The listing builds one solid part. Answer for the finished solid, in the listing's coordinates (mm). Face numbers are marked on the shaded views. Coordinates: 2 decimals unless noted, no trailing zeros. Order: outer loops, then holes, each group sorted by start corner. A loop starts at its lowest first (then second) coordinate and runs counter-clockwise, first axis right, second up.
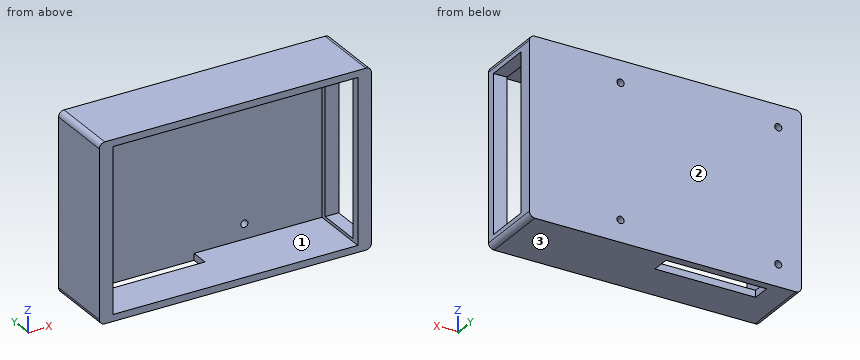
from build123d import *

# Parameters (mm, degrees)
SKETCH1_W           = 100
SKETCH1_H           = 65
BOSS_EXTRUDE2_DEPTH = 25
SKETCH1_5_W         = 90
SKETCH1_5_H         = 60
CUT_EXTRUDE1_DEPTH  = 22
SKETCH3_R           = 1.3
CUT_EXTRUDE2_DEPTH  = 18
FILLET2_R           = 2
FILLET3_R           = 2
FILLET4_R           = 2
FILLET5_R           = 2
SKETCH5_W           = 37
SKETCH5_H           = 6.720639237
CUT_EXTRUDE3_DEPTH  = 10
SKETCH6_W           = 57.574734681
SKETCH6_H           = 17
CUT_EXTRUDE4_DEPTH  = 10


with BuildPart() as part:
    # Sketch1 → Boss-Extrude2 (new body)
    with BuildSketch(Plane(origin=(0, 0, 0), x_dir=(1, 0, 0), z_dir=(0, 1, 0))):
        Rectangle(SKETCH1_W, SKETCH1_H)
    extrude(amount=BOSS_EXTRUDE2_DEPTH)

    # Sketch1_5 → Cut-Extrude1 (cut)
    with BuildSketch(Plane(origin=(0, 0, 0), x_dir=(1, 0, 0), z_dir=(0, 1, 0))):
        Rectangle(SKETCH1_5_W, SKETCH1_5_H)
    extrude(amount=CUT_EXTRUDE1_DEPTH, mode=Mode.SUBTRACT)

    # Sketch3 → Cut-Extrude2 (cut)
    with BuildSketch(Plane.XZ.offset(-22)):
        with Locations(Location((-41.5, 24.5, 0), (0, 0, 270))):
            Circle(SKETCH3_R)
        with Locations(Location((-41.5, -24.5, 0), (0, 0, 270))):
            Circle(SKETCH3_R)
        with Locations(Location((16.5, -24.5, 0), (0, 0, 270))):
            Circle(SKETCH3_R)
        with Locations(Location((16.5, 24.5, 0), (0, 0, 270))):
            Circle(SKETCH3_R)
    extrude(amount=-CUT_EXTRUDE2_DEPTH, mode=Mode.SUBTRACT)

    # Fillet2
    fillet2_edges = [part.edges().sort_by_distance(p)[0] for p in [
        (50, 12.5, 32.5),
    ]]
    fillet(fillet2_edges, radius=FILLET2_R)

    # Fillet3
    fillet3_edges = [part.edges().sort_by_distance(p)[0] for p in [
        (-50, 12.5, 32.5),
    ]]
    fillet(fillet3_edges, radius=FILLET3_R)

    # Fillet4
    fillet4_edges = [part.edges().sort_by_distance(p)[0] for p in [
        (-50, 12.5, -32.5),
    ]]
    fillet(fillet4_edges, radius=FILLET4_R)

    # Fillet5
    fillet5_edges = [part.edges().sort_by_distance(p)[0] for p in [
        (50, 12.5, -32.5),
    ]]
    fillet(fillet5_edges, radius=FILLET5_R)

    # Sketch5 → Cut-Extrude3 (cut)
    with BuildSketch(Plane(origin=(0, 0, -32.5), x_dir=(-1, 0, 0), z_dir=(0, 0, -1))):
        with Locations((20.5, 18.639680381)):
            Rectangle(SKETCH5_W, SKETCH5_H)
    extrude(amount=-CUT_EXTRUDE3_DEPTH, mode=Mode.SUBTRACT)

    # Sketch6 → Cut-Extrude4 (cut)
    with BuildSketch(Plane(origin=(50, 0, 0), x_dir=(0, 0, -1), z_dir=(1, 0, 0))):
        with Locations((0.07362498, 11.5)):
            Rectangle(SKETCH6_W, SKETCH6_H)
    extrude(amount=-CUT_EXTRUDE4_DEPTH, mode=Mode.SUBTRACT)


solid = part.part
(1) Find section C-C on x = -8.5. Determine the outline of the cut face in (y, z).
(2) Find section D-D on y = 10. Determine the outline of the cut face in (x, z), then the cut area to 3 significant figures.
(3) Find section A-A on z = 19.5. Determine the outline of the cut face in (x, y), then the cut area to 3 significant figures.
(4) The mould has two halves that part along Z. Classify the marked faces 1, 2 and 3: pulls with the +Z half, pulls with the -Z half, needs draft (parallel to the pull), parting line crosses it, or undercut.
(5) Find the intervals of material crossed by probe 1 along X at (y, z) = (23.7, -24.5); probe 2 along Z at (x, y) = (5, 13.75); probe 3 along X at (y, z) = (2.75, 20), in increasing order.
(6) Find section B-B on x = 16.5. Determine the outline of the cut face in (y, z).
(7) Given pin 1 Ø2.5 at (x, z) = (16.5, -24.5) entering from -Y; pin 2 Ø3.5 at (x, z) = (-41.5, 24.5) entering from -Y; pin 3 Ø6.5 at (y, z) = (11.5, 15) entering from +X; pin 4 Ø6 at (y, z) = (18, 15) entering from +X, each flat-ended and moving along its own axis, determine where each tip first touches the part or whether it passes through.
Resolved:
1. outline: (0, -32.5) - (15.28, -32.5) - (15.28, -30) - (0, -30) - close; (0, 30) - (22, 30) - (22, -32.5) - (25, -32.5) - (25, 32.5) - (0, 32.5) - close
2. outline: (-50, -30.5) arc R2 ccw to (-48, -32.5) - (48, -32.5) arc R2 ccw to (50, -30.5) - (50, -28.86) - (45, -28.86) - (45, -30) - (-45, -30) - (-45, 30) - (45, 30) - (45, 28.71) - (50, 28.71) - (50, 30.5) arc R2 ccw to (48, 32.5) - (-48, 32.5) arc R2 ccw to (-50, 30.5) - close
2. area: 809 mm2
3. outline: (-50, 0) - (-45, 0) - (-45, 22) - (45, 22) - (45, 20) - (50, 20) - (50, 25) - (-50, 25) - close; (45, 0) - (50, 0) - (50, 3) - (45, 3) - close
3. area: 435 mm2
4. face 1: undercut
4. face 2: needs draft
4. face 3: pulls with the -Z half
5. probe 1: x = -50 to -42.8, -40.2 to 15.2, 17.8 to 50
5. probe 2: z = -32.5 to -30, 30 to 32.5
5. probe 3: x = -50 to -45, 45 to 50
6. outline: (0, -32.5) - (25, -32.5) - (25, -25.8) - (22, -25.8) - (22, -30) - (0, -30) - close; (0, 30) - (22, 30) - (22, 25.8) - (25, 25.8) - (25, 32.5) - (0, 32.5) - close; (22, -23.2) - (25, -23.2) - (25, 23.2) - (22, 23.2) - close
7. pin 1: passes through
7. pin 2: stops at y = 22
7. pin 3: stops at x = -45
7. pin 4: stops at x = 50
